Source: three-view drawing plus pictorial views. Frame: mm from the lowest corner of the part. A direction names the side the tool comes from. Give positions to 0.01 mm unless a question says otherwise; leave off trailing zeros. Loops run counter-clockwise (first coordinate to the right, second up) from the corner with the lowest first, then second, coordinate; pieces in that order, holes last. Notation, with made-up numbers: M 72,-22 L 124,-22 A30 ccw 124,1 Z; hole C 2,-5 d10. An arc over 180 degrees is marked long. Answer as a JSON object with one key per item and string values. Group by question number.
1) Section query C-C on y = 5.5. Return loops of the section in (x, z).
2) Section query D-D on x = 50. Return loops of the section in (y, z), plus the area to 3 significant figures.
3) First-contact query: P1, Ø10, axis at y = 11, z = 18.5, coming from the +X side; P2, Ø5, axis at x = 13.5, z = 41, coming from the +Y side; P3, Ø4, axis at x = 38.75, z = 46.99, coming from the +Y side. Flat tips, straight axial feed; report the tip coordinate or a pass-through.
4) Section query A-A on z = 26.5. Count the separate pieces of the cut face and the enclosed holes in it, plus the area to 3 significant figures.
5) Access query for the marked faces 1 and 2. Directions: +Z, -Z, +X, -X, +Y, -Y. A direction counts if a zero-diameter tool reaches every point of the face in a straight line with its end or side. Return the directions, or none.
6) Ray query, L1, parallel to Y at x = 24, z = 33.5; L2, parallel to Y at x = 42.5, z = 36; L3, parallel to X at y = 27.5, z = 30.5 (1 decimal). Return the intervals inside material, ascending.
7) Section query B-B on x = 27.5. Return loops of the section in (y, z).
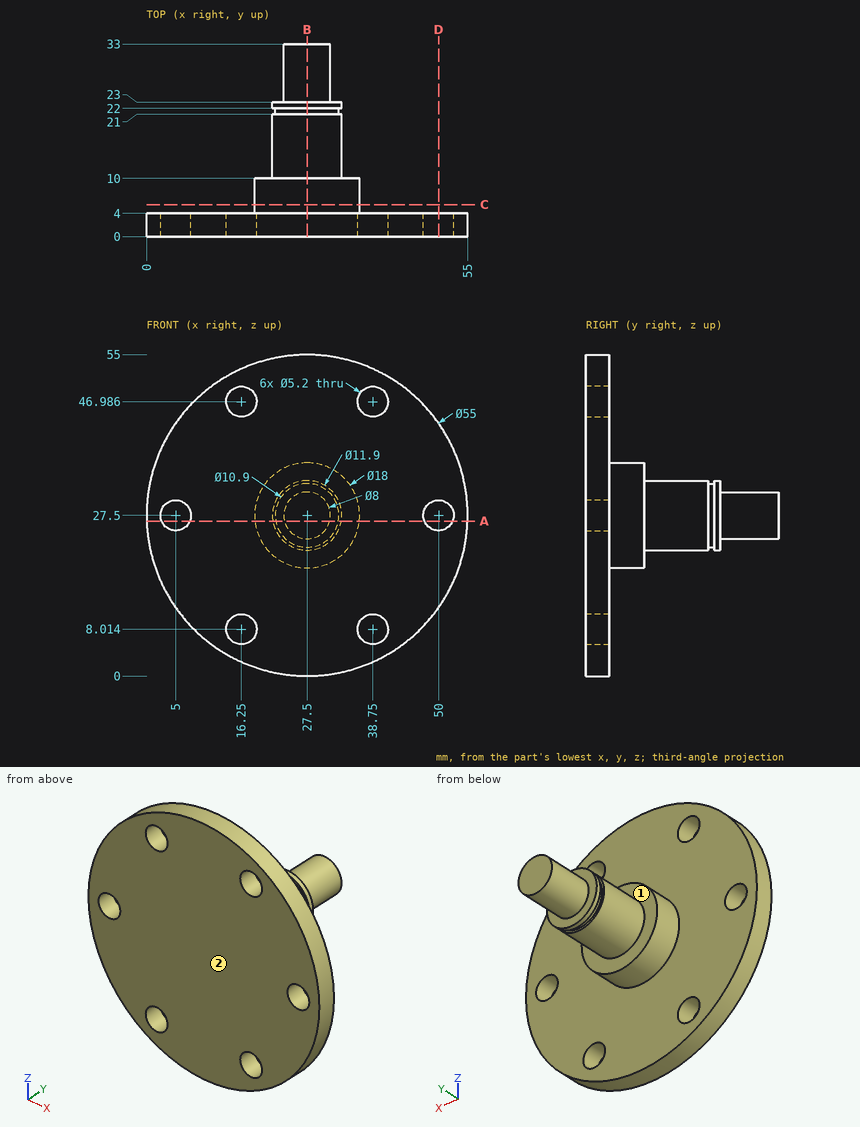
Output:
{
 "1": {"outline": "C 27.5,27.5 d18"},
 "2": {"outline": "M 0,11.69 L 4,11.69 L 4,24.9 L 0,24.9 Z; M 0,30.1 L 4,30.1 L 4,43.31 L 0,43.31 Z", "area": "106 mm^2"},
 "3": {"P1": "stops at x = 35.51", "P2": "stops at y = 4", "P3": "passes through"},
 "4": {"separate pieces": "3", "enclosed holes": "0", "area": "518 mm^2"},
 "5": {"face 1": "+Y", "face 2": "+Z, -Z, +X, -X, -Y"},
 "6": {"L1": "y = 0 to 10", "L2": "y = 0 to 4", "L3": "x = 24.9 to 30.1"},
 "7": {"outline": "M 0,0 L 4,0 L 4,18.5 L 10,18.5 L 10,21.55 L 21,21.55 L 21,22.05 L 22,22.05 L 22,21.55 L 23,21.55 L 23,23.5 L 33,23.5 L 33,31.5 L 23,31.5 L 23,33.45 L 22,33.45 L 22,32.95 L 21,32.95 L 21,33.45 L 10,33.45 L 10,36.5 L 4,36.5 L 4,55 L 0,55 Z"}
}
